```python
from build123d import *

# Parameters (mm, degrees)
SKETCH1_R               = 5.2
SKETCH1_R_2             = 4.65
BOSS_EXTRUDE1_DEPTH     = 121.35
SKETCH2_R               = 6.32
SKETCH2_R_2             = 4.65
BOSS_EXTRUDE2_DEPTH     = 15.8
SKETCH4_R               = 11.4
SKETCH4_R_2             = 10.4
BOSS_EXTRUDE3_DEPTH     = 19.9
BOSS_EXTRUDE4_DEPTH     = 6.5
CUT_EXTRUDE1_DEPTH      = 4.8
FILLET2_R               = 10
SKETCH8_R               = 4.65
CUT_EXTRUDE2_DEPTH      = 159.003069696
CUT_EXTRUDE2_DEPTH_BACK = 159.003069696
FILLET3_R               = 5
FILLET4_R               = 5


with BuildPart() as part:
    # Sketch1 → Boss-Extrude1 (new body)
    with BuildSketch(Plane(origin=(0, 0, 0), x_dir=(1, 0, 0), z_dir=(0, 1, 0))):
        with Locations(Location((0, 0, 0), (0, 0, 270))):
            Circle(SKETCH1_R)
        with Locations(Location((0, 0, 0), (0, 0, 270))):
            Circle(SKETCH1_R_2, mode=Mode.SUBTRACT)
    extrude(amount=BOSS_EXTRUDE1_DEPTH)

    # Sketch2 → Boss-Extrude2 (add)
    with BuildSketch(Plane(origin=(0, 121.35, 0), x_dir=(1, 0, 0), z_dir=(0, 1, 0))):
        with Locations(Location((0, 0, 0), (0, 0, 270))):
            Circle(SKETCH2_R)
        with Locations(Location((0, 0, 0), (0, 0, 270))):
            Circle(SKETCH2_R_2, mode=Mode.SUBTRACT)
    extrude(amount=-BOSS_EXTRUDE2_DEPTH)

    # Sketch3 → Revolve1 (revolve)
    with BuildSketch(Plane.XY, mode=Mode.PRIVATE) as revolve1_sk:
        Polygon((-6.32, 121.35), (-11.4, 135), (-10.4, 135), (-4.65, 121.35), align=None)
    revolve(revolve1_sk.sketch.rotate(Axis((0, 121.35, 0), (0, -1, 0)), 270), axis=Axis((0, 121.35, 0), (0, -1, 0)))

    # Sketch4 → Boss-Extrude3 (add)
    with BuildSketch(Plane(origin=(0, 135, 0), x_dir=(1, 0, 0), z_dir=(0, 1, 0))):
        with Locations(Location((0, 0, 0), (0, 0, 90))):
            Circle(SKETCH4_R)
        with Locations(Location((0, 0, 0), (0, 0, 90))):
            Circle(SKETCH4_R_2, mode=Mode.SUBTRACT)
    extrude(amount=BOSS_EXTRUDE3_DEPTH)

    # Fillet2
    fillet2_edges = [part.edges().sort_by_distance(p)[0] for p in [
        (-11.4, 135, 0),
    ]]
    fillet(fillet2_edges, radius=FILLET2_R)


with BuildPart() as body_2:
    # Sketch6 → Boss-Extrude4 (new body)
    with BuildSketch(Plane.XY.offset(6.32)):
        Polygon((-10.3, 105.55), (10.3, 105.55), (29, 139.89), (29, 145.55), (22.7, 145.55), (22.7, 139.89), (12.603960396, 121.35), (-12.603960396, 121.35), (-22.7, 139.89), (-22.7, 145.55), (-29, 145.55), (-29, 139.89), align=None)
    extrude(amount=-BOSS_EXTRUDE4_DEPTH)

    # Sketch7 → Cut-Extrude1 (cut)
    with BuildSketch(Plane.XY.offset(6.32)):
        with BuildLine():
            Line((8.3, 119.257622479), (12.456070352, 119.257622479))
            ThreePointArc((12.456070352, 119.257622479), (13.745534607, 118.523965702), (13.773633276, 117.04066506))
            Line((13.773633276, 117.04066506), (9.534103268, 109.249619999))
            ThreePointArc((9.534103268, 109.249619999), (8.982883567, 108.677113163), (8.216540343, 108.466577418))
            Line((8.216540343, 108.466577418), (7.8, 108.466577418))
            ThreePointArc((7.8, 108.466577418), (7.092893219, 108.759470637), (6.8, 109.466577418))
            Line((6.8, 109.466577418), (6.8, 117.757622479))
            ThreePointArc((6.8, 117.757622479), (7.239339828, 118.81828265), (8.3, 119.257622479))
        make_face()
        with BuildLine():
            Line((-15.248616144, 123.653554953), (-23.653367428, 139.099086851))
            ThreePointArc((-23.653367428, 139.099086851), (-25.757025654, 139.720102373), (-26.378041176, 137.616444147))
            Line((-26.378041176, 137.616444147), (-17.973289892, 122.170912249))
            ThreePointArc((-17.973289892, 122.170912249), (-15.869631666, 121.549896727), (-15.248616144, 123.653554953))
        make_face()
        with BuildLine():
            Line((15.248616144, 123.653554953), (23.653367428, 139.099086851))
            ThreePointArc((23.653367428, 139.099086851), (25.757025654, 139.720102373), (26.378041176, 137.616444147))
            Line((26.378041176, 137.616444147), (17.973289892, 122.170912249))
            ThreePointArc((17.973289892, 122.170912249), (15.869631666, 121.549896727), (15.248616144, 123.653554953))
        make_face()
        with BuildLine():
            Line((-8.216540343, 108.466577418), (-7.8, 108.466577418))
            ThreePointArc((-7.8, 108.466577418), (-7.092893219, 108.759470637), (-6.8, 109.466577418))
            Line((-6.8, 109.466577418), (-6.8, 117.757622479))
            ThreePointArc((-6.8, 117.757622479), (-7.239339828, 118.81828265), (-8.3, 119.257622479))
            Line((-8.3, 119.257622479), (-12.456070352, 119.257622479))
            ThreePointArc((-12.456070352, 119.257622479), (-13.745534607, 118.523965702), (-13.773633276, 117.04066506))
            Line((-13.773633276, 117.04066506), (-9.534103268, 109.249619999))
            ThreePointArc((-9.534103268, 109.249619999), (-8.982883567, 108.677113163), (-8.216540343, 108.466577418))
        make_face()
    extrude(amount=-CUT_EXTRUDE1_DEPTH, mode=Mode.SUBTRACT)

    # Sketch8 → Cut-Extrude2 (cut, two sides)
    with BuildSketch(Plane(origin=(0, 0, 0), x_dir=(1, 0, 0), z_dir=(0, 1, 0))) as cut_extrude2_sk:
        with Locations(Location((0, 0, 0), (0, 0, 270))):
            Circle(SKETCH8_R)
    extrude(amount=CUT_EXTRUDE2_DEPTH, mode=Mode.SUBTRACT)
    extrude(cut_extrude2_sk.sketch, amount=-CUT_EXTRUDE2_DEPTH_BACK, mode=Mode.SUBTRACT)

    # Combine1: union part
    add(part.part)

    # Fillet3
    fillet3_edges = [body_2.edges().sort_by_distance(p)[0] for p in [
        (-6.317436189, 113.45, -0.18),
    ]]
    fillet(fillet3_edges, radius=FILLET3_R)

    # Fillet4
    fillet4_edges = [body_2.edges().sort_by_distance(p)[0] for p in [
        (6.317436189, 113.45, -0.18),
    ]]
    fillet(fillet4_edges, radius=FILLET4_R)


solid = body_2.part
```
Part model, mm, in its own coordinate system. A direction names the side the tool comes from. Round coordinates to 2 decimals unless told otherwise and drop trailing zeros. Write each loop counter-clockwise with the first axis right and the second up, starting at its lowest first coordinate (ties: lowest second). Pieces come first, ordered by that corner, then holes. Notation, with made-up numbers: (23, -16.75) -> (73, -16.75) arc R7 ccw to (73, -11.75) -> close; hole circle Ø1 at (1.5, 72.5). An arc over 180 degrees is marked (long way). Return JSON: item names as keys, results as strings. Group by question number.
Q1. Which spindle directions (+Z, -Z, +X, -X, +Y, -Y) get a long thin tool onto all of the face, cutting with end or side? Do faces 4 (the flat face through (29, 143, 3)), 5 (the flat face through (17.723, 130.75, 3.116)), 6 (the flat face through (-22.234, 130.002, 3.954)), 7 (the cylindrical face through (7.494, 113.561, -0.892)), 8 (the flat face through (-29, 143, 3)). Say none if no direction does.
Q2. Probe L1, parallel to X at y = 143.5, z = 0; L2, parallel to X at y = 149.75, z = 0; L3, parallel to X at y = 70, z = 0. List the from-to ranges inside material, lowest first. Write a range as [from, to].
Q3. Pin check, flat tips, straight feed: pin 1 (10 mm diameter, centred on x = -8.5, z = 2, fed in from +Y); pin 2 (0.5 mm diameter, centred on x = 8, z = 3.5, fed in from +Y); pin 3 (4 mm diameter, centred on x = 16.5, z = -1.5, fed in from +Y); pin 4 (5 mm diameter, centred on x = 25.5, z = 4, fed in from +Y). Stop position of each tip, or through.
Q4. Mould opens along Y. For faces 1 (the flat face through (-26, 145.55, 3)), 2 (the conical face through (4.62, 124.76, -6.02)), 3 (the flat face through (-3, 0, -4)) say: pulls with the +Y half, pulls with the -Y half, needs draft (parallel to the pull), parting line crosses it, or undercut.
Q5. Saw through at C-C on y = 73.5. Write the cut outline in (x, z).
Q6. Saw through at A-A on y = 141.5. Write the cut outline in (x, z).
Q7. Saw through at B-B on x = 19.5. Write the cut outline in (y, z), plus the area to 3 significant figures.
Answer:
{
 "1": {"face 4": "+Z, -Z, +X, +Y, -Y", "face 5": "+Z, -Z, +Y", "face 6": "+Z", "face 7": "-Z, +X, -Y", "face 8": "+Z, -Z, -X, +Y, -Y"},
 "2": {"L1": "[-29, -22.7], [-11.4, -10.4], [10.4, 11.4], [22.7, 29]", "L2": "[-11.4, -10.4], [10.4, 11.4]", "L3": "[-5.2, -4.65], [4.65, 5.2]"},
 "3": {"pin 1": "y = 154.9", "pin 2": "y = 131.63", "pin 3": "y = 131.26", "pin 4": "y = 145.55"},
 "4": {"face 1": "pulls with the +Y half", "face 2": "undercut", "face 3": "pulls with the -Y half"},
 "5": {"outline": "circle Ø10.4 at (0, 0); hole circle Ø9.3 at (0, 0)"},
 "6": {"outline": "(-29, -0.18) -> (-22.7, -0.18) -> (-22.7, 6.32) -> (-29, 6.32) -> close; circle Ø22.8 at (0, 0); (22.7, -0.18) -> (29, -0.18) -> (29, 6.32) -> (22.7, 6.32) -> close; hole circle Ø20.8 at (0, 0)"},
 "7": {"outline": "(122.44, -0.18) -> (134.01, -0.18) -> (134.01, 6.32) -> (131.47, 6.32) -> (131.47, 1.52) -> (124.98, 1.52) -> (124.98, 6.32) -> (122.44, 6.32) -> close", "area": "44.0 mm2"}
}
